Could you check a few things on this model? Use its own coordinates, in mm. Face numbers are marked on the shaded views. A direction names the side the tool comes from. Round coordinates to 2 decimals unless told otherwise and drop trailing zeros. Write each loop counter-clockwise with the first axis right and the second up, starting at its lowest first coordinate (ties: lowest second). Pieces come first, ordered by that corner, then holes. Notation, with made-up numbers: (-11.5, 4.5) -> (43.5, 4.5) arc R17 cw to (43.5, 19.5) -> close; hole circle Ø6 at (50.25, -9). An arc over 180 degrees is marked (long way). Answer in a Markdown table with one row per item.
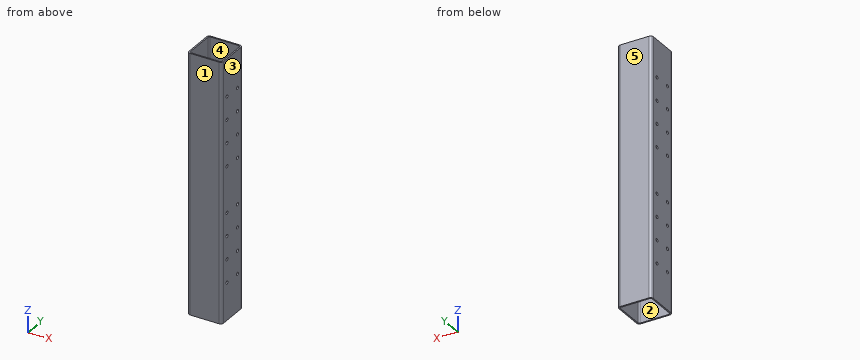
from build123d import *

# Parameters (mm, degrees)
BOSS_EXTRUDE1_DEPTH = 571.5
SKETCH2_R           = 6.985
CUT_EXTRUDE1_DEPTH  = 597.359329599


with BuildPart() as part:
    # Sketch1 → Boss-Extrude1 (new, symmetric)
    with BuildSketch(Plane.XY):
        with BuildLine():
            Line((-63.5, -76.2), (63.5, -76.2))
            ThreePointArc((63.5, -76.2), (72.480256121, -72.480256121), (76.2, -63.5))
            Line((76.2, -63.5), (76.2, 63.5))
            ThreePointArc((76.2, 63.5), (72.480256121, 72.480256121), (63.5, 76.2))
            Line((63.5, 76.2), (-63.5, 76.2))
            ThreePointArc((-63.5, 76.2), (-72.480256121, 72.480256121), (-76.2, 63.5))
            Line((-76.2, 63.5), (-76.2, -63.5))
            ThreePointArc((-76.2, -63.5), (-72.480256121, -72.480256121), (-63.5, -76.2))
        make_face()
        with BuildLine():
            Line((-63.5, 69.85), (63.5, 69.85))
            ThreePointArc((63.5, 69.85), (67.990128061, 67.990128061), (69.85, 63.5))
            Line((69.85, 63.5), (69.85, -63.5))
            ThreePointArc((69.85, -63.5), (67.990128061, -67.990128061), (63.5, -69.85))
            Line((63.5, -69.85), (-63.5, -69.85))
            ThreePointArc((-63.5, -69.85), (-67.990128061, -67.990128061), (-69.85, -63.5))
            Line((-69.85, -63.5), (-69.85, 63.5))
            ThreePointArc((-69.85, 63.5), (-67.990128061, 67.990128061), (-63.5, 69.85))
        make_face(mode=Mode.SUBTRACT)
    extrude(amount=BOSS_EXTRUDE1_DEPTH, both=True)

    # Sketch2 → Cut-Extrude1 (cut, through all)
    with BuildSketch(Plane.ZY.offset(76.2)):
        with Locations((-101.6, 38.1)):
            Circle(SKETCH2_R)
        with Locations((-203.2, 38.1)):
            Circle(SKETCH2_R)
        with Locations((-304.8, 38.1)):
            Circle(SKETCH2_R)
        with Locations((-304.8, -38.1)):
            Circle(SKETCH2_R)
        with Locations((-203.2, -38.1)):
            Circle(SKETCH2_R)
        with Locations((-101.6, -38.1)):
            Circle(SKETCH2_R)
        with Locations((101.6, -38.1)):
            Circle(SKETCH2_R)
        with Locations((203.2, -38.1)):
            Circle(SKETCH2_R)
        with Locations((304.8, -38.1)):
            Circle(SKETCH2_R)
        with Locations((304.8, 38.1)):
            Circle(SKETCH2_R)
        with Locations((203.2, 38.1)):
            Circle(SKETCH2_R)
        with Locations((101.6, 38.1)):
            Circle(SKETCH2_R)
        with Locations((-406.4, 38.1)):
            Circle(SKETCH2_R)
        with Locations((-406.4, -38.1)):
            Circle(SKETCH2_R)
        with Locations((406.4, -38.1)):
            Circle(SKETCH2_R)
        with Locations((406.4, 38.1)):
            Circle(SKETCH2_R)
    extrude(amount=-CUT_EXTRUDE1_DEPTH, mode=Mode.SUBTRACT)


solid = part.part
1) Thinking about a two-plate mould opening in Y: for the marked faces 3, 4 and 5, which applies, +Y half, -Y half, draft (parallel to the pull), parting line (faces both ways), or undercut?
Findings:
| item | result |
|---|---|
| face 3 | draft |
| face 4 | undercut |
| face 5 | +Y half |
2) For the marked faces 1 and 2, which set-ups out of +Z, -Z, +X, -X, +Y, -Y let a thin tool reach every point of the face, with its end or its side?
Findings:
| item | result |
|---|---|
| face 1 | +Z, -Z, +X, -X, -Y |
| face 2 | +Z, -Z |
3) Imagine slicing it at A-A, the plane x = 9.5. Please give me the cut outline in (y, z), plus the area to 3 significant figures.
Findings:
| item | result |
|---|---|
| outline | (-76.2, -571.5) -> (-69.85, -571.5) -> (-69.85, 571.5) -> (-76.2, 571.5) -> close; (69.85, -571.5) -> (76.2, -571.5) -> (76.2, 571.5) -> (69.85, 571.5) -> close |
| area | 14,500 mm^2 |
4) Imagine slicing it at B-B, the plane z = -162. Please give me the cut outline in (x, y).
Findings:
| item | result |
|---|---|
| outline | (-76.2, -63.5) arc R12.7 ccw to (-63.5, -76.2) -> (63.5, -76.2) arc R12.7 ccw to (76.2, -63.5) -> (76.2, 63.5) arc R12.7 ccw to (63.5, 76.2) -> (-63.5, 76.2) arc R12.7 ccw to (-76.2, 63.5) -> close; hole (-69.85, -63.5) arc R6.35 ccw to (-63.5, -69.85) -> (63.5, -69.85) arc R6.35 ccw to (69.85, -63.5) -> (69.85, 63.5) arc R6.35 ccw to (63.5, 69.85) -> (-63.5, 69.85) arc R6.35 ccw to (-69.85, 63.5) -> close |
5) For pin 1 (18 mm diameter, centred on y = -38.1, z = 101.6, fed in from +X), with a flat end and sliding along its axis, tell me the tip position at first contact or that it passes through.
Findings:
| item | result |
|---|---|
| pin 1 | stops at x = 76.2 |
6) Please list where these lines run through material, in increasing order: line 1 (Y direction, x = -74.5, z = 406.4) (3 decimals); line 2 (X direction, y = -19, z = -416).
Findings:
| item | result |
|---|---|
| line 1 | y = -69.847 to -45.085, -31.115 to 31.115, 45.085 to 69.847 |
| line 2 | x = -76.2 to -69.85, 69.85 to 76.2 |
